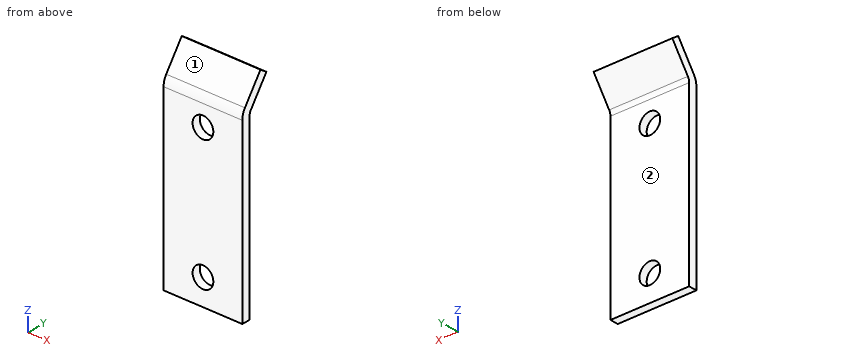
```python
from build123d import *

# Parameters (mm, degrees)
F1_DEPTH = 76
F2_R     = 10
F3_DEPTH = 8.001


with BuildPart() as f1:
    # F0 (on Right) → F1 (new body)
    with BuildSketch(Plane.YZ):
        with BuildLine():
            Line((0, 170), (0, 0))
            Line((0, 0), (8, 0))
            Line((8, 0), (8, 170))
            ThreePointArc((8, 170), (8.370264, 172.405646), (9.446784, 174.588611))
            Line((9.446784, 174.588611), (26.654077, 199.163173))
            Line((26.654077, 199.163173), (20.10086, 203.751784))
            Line((20.10086, 203.751784), (2.893567, 179.177223))
            ThreePointArc((2.893567, 179.177223), (0.740529, 174.811293), (0, 170))
        make_face()
    extrude(amount=F1_DEPTH)

    # F2 (on face) → F3 (cut, through all)
    with BuildSketch(Plane(origin=(0, 8, 0), x_dir=(-1, 0, 0), z_dir=(0, 1, 0))):
        with Locations((-38, 150)):
            Circle(F2_R)
        with Locations((-38, 25)):
            Circle(F2_R)
    extrude(amount=-F3_DEPTH, mode=Mode.SUBTRACT)


solid = f1.part
```
Can you work these out from the model? Positions are in its coordinate system, mm. Face numbers are marked on the shaded views. A direction names the side the tool comes from. Round coordinates to 2 decimals unless told otherwise and drop trailing zeros. Loops run counter-clockwise (first coordinate to the right, second up) from the corner with the lowest first, then second, coordinate; pieces in that order, holes last.
Item 1: Which directions (+Z, -Z, +X, -X, +Y, -Y) give clear straight access to the entire face, cutting with the end or side of a thin tool? Please do the marked faces 1 and 2.
Item 2: Will these pins go through, and if not, where does the flat tip stop? pin 1 Ø1.5 at (x, y) = (54, 17) entering from -Z; pin 2 Ø6 at (x, y) = (19, 5.5) entering from +Z; pin 3 Ø2 at (x, y) = (54.5, 19) entering from -Z.
Item 3: Please list where these lines run through material, in increasing order: L1, parallel to Z at x = 38, y = 5.5; L2, parallel to Z at x = 38, y = 4.25; L3, parallel to Y at x = 57, z = 33.5.
Item 4: Suppose I cut it at C-C, the plane x = 63. Write out the boundary of the cut face in (y, z).
Item 5: Suppose I cut it at D-D, the plane z = 128.5. Write out the boundary of the cut face in (x, y).
Item 6: Suppose I cut it at A-A, the plane x = 38. Write out the boundary of the cut face in (y, z).
Item 7: Suppose I cut it at B-B, the plane z = 150. Write out the boundary of the cut face in (x, y).
Reported:
1. face 1: +Z, +X, -X, -Y
1. face 2: -Z, +X, -X, +Y
2. pin 1: stops at z = 184.3
2. pin 2: stops at z = 187.18
2. pin 3: stops at z = 186.8
3. L1: z = 0 to 15, 35 to 140, 160 to 182.9
3. L2: z = 0 to 15, 35 to 140, 160 to 181.11
3. L3: y = 0 to 8
4. outline: (0, 0) - (8, 0) - (8, 170) arc R8 cw to (9.45, 174.59) - (26.65, 199.16) - (20.1, 203.75) - (2.89, 179.18) arc R16 ccw to (0, 170) - close
5. outline: (0, 0) - (76, 0) - (76, 8) - (0, 8) - close
6. outline: (0, 0) - (8, 0) - (8, 15) - (0, 15) - close; (0, 35) - (8, 35) - (8, 140) - (0, 140) - close; (0, 160) - (8, 160) - (8, 170) arc R8 cw to (9.45, 174.59) - (26.65, 199.16) - (20.1, 203.75) - (2.89, 179.18) arc R16 ccw to (0, 170) - close
7. outline: (0, 0) - (28, 0) - (28, 8) - (0, 8) - close; (48, 0) - (76, 0) - (76, 8) - (48, 8) - close
